```python
from build123d import *

# Parameters (mm, degrees)
SKETCH1_R                = 9.5
BOSS_EXTRUDE1_DEPTH      = 3
BOSS_EXTRUDE1_2_DEPTH    = 3
BOSS_EXTRUDE2_DEPTH      = 5
BOSS_EXTRUDE3_DEPTH      = 15.5
BOSS_EXTRUDE3_DEPTH_BACK = 1.5
BOSS_EXTRUDE4_DEPTH      = 8.5
BOSS_EXTRUDE4_DEPTH_BACK = 1.5
SKETCH1_5_R              = 10
SKETCH1_5_R_2            = 2.5
BOSS_EXTRUDE5_DEPTH      = 8.5
BOSS_EXTRUDE5_DEPTH_BACK = 1.5
SKETCH1_6_R              = 2.5
BOSS_EXTRUDE6_DEPTH      = 15.5
BOSS_EXTRUDE6_DEPTH_BACK = 1.5
SKETCH1_7_R              = 20
SKETCH1_7_R_2            = 15.5
CUT_EXTRUDE1_REACH       = 89.409
SKETCH8_W                = 16.25
SKETCH8_H                = 1.075
BOSS_EXTRUDE7_START      = 1.5
BOSS_EXTRUDE7_DEPTH      = 1.5


with BuildPart() as part:
    # Sketch1 → Boss-Extrude1 (new body)
    with BuildSketch(Plane(origin=(0, 0, 0), x_dir=(1, 0, 0), z_dir=(0, 1, 0))):
        with BuildLine():
            ThreePointArc((-30.156865167, -2.5), (-33.272749334, -10.963534337), (-39.790126097, -17.197629921))
            ThreePointArc((-39.790126097, -17.197629921), (-41.249487369, -19.543048034), (-40.173039204, -22.087056839))
            Line((-40.173039204, -22.087056839), (-14.241082593, -35.680284508))
            ThreePointArc((-14.241082593, -35.680284508), (-11.504148883, -36.255537388), (-9.482068, -34.323463137))
            ThreePointArc((-9.482068, -34.323463137), (-1.352594655, -27.591897876), (8.28370035, -31.898187034))
            ThreePointArc((8.28370035, -31.898187034), (10.418414325, -33.197109967), (12.796233312, -32.428877315))
            Line((12.796233312, -32.428877315), (28.974944097, -17.384928273))
            ThreePointArc((28.974944097, -17.384928273), (29.945946241, -15.076495792), (28.827477371, -12.835796554))
            ThreePointArc((28.827477371, -12.835796554), (27.255378579, -11.246023539), (26.082304527, -9.342665949))
            ThreePointArc((26.082304527, -9.342665949), (24.834057729, -6.000240645), (24.142507006, -2.5))
            Line((24.142507006, -2.5), (-30.156865167, -2.5))
        make_face()
        with Locations(Location((1, -14.5, 0), (0, 0, 270))):
            Circle(SKETCH1_R, mode=Mode.SUBTRACT)
    extrude(amount=BOSS_EXTRUDE1_DEPTH)



with BuildPart() as body_2:
    # Sketch1 → Boss-Extrude1 2 (new body)
    with BuildSketch(Plane(origin=(0, 0, 0), x_dir=(1, 0, 0), z_dir=(0, 1, 0))):
        with BuildLine():
            ThreePointArc((8.284210438, 31.898941402), (-1.363739049, 27.593425627), (-9.489477618, 34.345667337))
            ThreePointArc((-9.489477618, 34.345667337), (-11.573635866, 36.300800208), (-14.349825716, 35.623282637))
            Line((-14.349825716, 35.623282637), (-40.302516761, 22.019186222))
            ThreePointArc((-40.302516761, 22.019186222), (-41.273789994, 19.493443338), (-39.816532128, 17.213279237))
            ThreePointArc((-39.816532128, 17.213279237), (-33.281167386, 10.97636716), (-30.156865167, 2.5))
            Line((-30.156865167, 2.5), (24.142507006, 2.5))
            ThreePointArc((24.142507006, 2.5), (24.834057729, 6.000240645), (26.082304527, 9.342665949))
            ThreePointArc((26.082304527, 9.342665949), (27.255658523, 11.24637974), (28.828183508, 12.836364321))
            ThreePointArc((28.828183508, 12.836364321), (29.944640188, 15.02344116), (29.053717415, 17.311680053))
            Line((29.053717415, 17.311680053), (12.87474854, 32.355869082))
            ThreePointArc((12.87474854, 32.355869082), (10.472331387, 33.203871974), (8.284210438, 31.898941402))
        make_face()
        with Locations(Location((1, 14.5, 0), (0, 0, 270))):
            Circle(SKETCH1_R, mode=Mode.SUBTRACT)
    extrude(amount=BOSS_EXTRUDE1_2_DEPTH)


with BuildPart() as part_1:
    add(part.part)

    add(body_2.part)  # Boss-Extrude2 merges body 2
    # Sketch1_3 → Boss-Extrude2 (add)
    with BuildSketch(Plane(origin=(0, 0, 0), x_dir=(1, 0, 0), z_dir=(0, 1, 0))):
        with BuildLine():
            ThreePointArc((-39.790126097, -17.197629921), (-49.47057805, -19.992991582), (-59.285404172, -17.713872229))
            Line((-59.285404172, -17.713872229), (-4.642702086, -46.356936115))
            ThreePointArc((-4.642702086, -46.356936115), (-9.277844603, -41.231165974), (-9.482068, -34.323463137))
            ThreePointArc((-9.482068, -34.323463137), (-11.504148883, -36.255537388), (-14.241082593, -35.680284508))
            Line((-14.241082593, -35.680284508), (-40.173039204, -22.087056839))
            ThreePointArc((-40.173039204, -22.087056839), (-41.249487369, -19.543048034), (-39.790126097, -17.197629921))
        make_face()
        with BuildLine():
            ThreePointArc((10, -37.5), (9.167764123, -41.494008136), (6.809579802, -44.823224898))
            Line((6.809579802, -44.823224898), (41.707436105, -12.373076129))
            ThreePointArc((41.707436105, -12.373076129), (35.353639159, -15.0033493), (28.827477371, -12.835796554))
            ThreePointArc((28.827477371, -12.835796554), (29.945946241, -15.076495792), (28.974944097, -17.384928273))
            Line((28.974944097, -17.384928273), (12.796233312, -32.428877315))
            ThreePointArc((12.796233312, -32.428877315), (10.418414325, -33.197109967), (8.28370035, -31.898187034))
            ThreePointArc((8.28370035, -31.898187034), (9.561302304, -34.570580561), (10, -37.5))
        make_face()
        with BuildLine():
            Line((41.707436105, 12.373076129), (6.809579802, 44.823224898))
            ThreePointArc((6.809579802, 44.823224898), (9.167764123, 41.494008136), (10, 37.5))
            ThreePointArc((10, 37.5), (9.561435676, 34.571015908), (8.284210438, 31.898941402))
            ThreePointArc((8.284210438, 31.898941402), (10.472331387, 33.203871974), (12.87474854, 32.355869082))
            Line((12.87474854, 32.355869082), (29.053717415, 17.311680053))
            ThreePointArc((29.053717415, 17.311680053), (29.944640188, 15.02344116), (28.828183508, 12.836364321))
            ThreePointArc((28.828183508, 12.836364321), (35.354091909, 15.003333024), (41.707436105, 12.373076129))
        make_face()
        with BuildLine():
            ThreePointArc((-9.489477618, 34.345667337), (-9.273471314, 41.242022153), (-4.642702086, 46.356936115))
            Line((-4.642702086, 46.356936115), (-59.285404172, 17.713872229))
            ThreePointArc((-59.285404172, 17.713872229), (-49.4859203, 19.99339196), (-39.816532128, 17.213279237))
            ThreePointArc((-39.816532128, 17.213279237), (-41.273789994, 19.493443338), (-40.302516761, 22.019186222))
            Line((-40.302516761, 22.019186222), (-14.349825716, 35.623282637))
            ThreePointArc((-14.349825716, 35.623282637), (-11.573635866, 36.300800208), (-9.489477618, 34.345667337))
        make_face()
    extrude(amount=BOSS_EXTRUDE2_DEPTH)

    # Sketch1_4 → Boss-Extrude3 (add, two sides: drawn at the far end of the back side and taken through both)
    with BuildSketch(Plane(origin=(0, 0, 0), x_dir=(1, 0, 0), z_dir=(0, 1, 0)).offset(-BOSS_EXTRUDE3_DEPTH_BACK)):
        with BuildLine():
            Line((24.142507006, 2.5), (-30.156865167, 2.5))
            ThreePointArc((-30.156865167, 2.5), (-30.039254815, 1.252458251), (-30, 0))
            ThreePointArc((-30, 0), (-30.039254815, -1.252458251), (-30.156865167, -2.5))
            Line((-30.156865167, -2.5), (24.142507006, -2.5))
            ThreePointArc((24.142507006, -2.5), (24, 0), (24.142507006, 2.5))
        make_face()
    extrude(amount=BOSS_EXTRUDE3_DEPTH + BOSS_EXTRUDE3_DEPTH_BACK)

    # Sketch1_5 → Boss-Extrude4 (add, two sides: drawn at the far end of the back side and taken through both)
    # profile 1 of 2: a face of its own
    with BuildSketch(Plane(origin=(0, 0, 0), x_dir=(1, 0, 0), z_dir=(0, 1, 0)).offset(-BOSS_EXTRUDE4_DEPTH_BACK)):
        with Locations(Location((0, -37.5, 0), (0, 0, 270))):
            Circle(SKETCH1_5_R)
        with Locations(Location((0, -37.5, 0), (0, 0, 270))):
            Circle(SKETCH1_5_R_2, mode=Mode.SUBTRACT)
    # profile 2 of 2: a face of its own
    with BuildSketch(Plane(origin=(0, 0, 0), x_dir=(1, 0, 0), z_dir=(0, 1, 0)).offset(-BOSS_EXTRUDE4_DEPTH_BACK)):
        with Locations(Location((0, 37.5, 0), (0, 0, 270))):
            Circle(SKETCH1_5_R)
        with Locations(Location((0, 37.5, 0), (0, 0, 270))):
            Circle(SKETCH1_5_R_2, mode=Mode.SUBTRACT)
    extrude(amount=BOSS_EXTRUDE4_DEPTH + BOSS_EXTRUDE4_DEPTH_BACK)

    # Sketch1_6 → Boss-Extrude5 (add, two sides: drawn at the far end of the back side and taken through both)
    with BuildSketch(Plane(origin=(0, 0, 0), x_dir=(1, 0, 0), z_dir=(0, 1, 0)).offset(-BOSS_EXTRUDE5_DEPTH_BACK)):
        with BuildLine():
            ThreePointArc((26.082304527, -9.342665949), (35, -15.009699604), (43.917695473, -9.342665949))
            ThreePointArc((43.917695473, -9.342665949), (46, 0), (43.917695473, 9.342665949))
            ThreePointArc((43.917695473, 9.342665949), (35, 15.009699604), (26.082304527, 9.342665949))
            ThreePointArc((26.082304527, 9.342665949), (24, 0), (26.082304527, -9.342665949))
        make_face()
        with Locations(Location((35, 0, 0), (0, 0, 270))):
            Circle(SKETCH1_6_R, mode=Mode.SUBTRACT)
    extrude(amount=BOSS_EXTRUDE5_DEPTH + BOSS_EXTRUDE5_DEPTH_BACK)

    # Sketch1_7 → Boss-Extrude6 (add, two sides: drawn at the far end of the back side and taken through both)
    with BuildSketch(Plane(origin=(0, 0, 0), x_dir=(1, 0, 0), z_dir=(0, 1, 0)).offset(-BOSS_EXTRUDE6_DEPTH_BACK)):
        with Locations((-50, 0)):
            Circle(SKETCH1_7_R)
        with Locations(Location((-50, 0, 0), (0, 0, 270))):
            Circle(SKETCH1_7_R_2, mode=Mode.SUBTRACT)
    extrude(amount=BOSS_EXTRUDE6_DEPTH + BOSS_EXTRUDE6_DEPTH_BACK)

    # Sketch3 → Cut-Extrude1 (cut, up to next)
    with BuildSketch(Plane.XY.offset(2.5), mode=Mode.PRIVATE) as cut_extrude1_sk1:
        Polygon((-30.156865167, 15.5), (24.142507006, 8.5), (24.142507006, 15.5), align=None)
    cut_extrude1_tool1 = extrude(cut_extrude1_sk1.sketch, amount=-CUT_EXTRUDE1_REACH, mode=Mode.PRIVATE) & part_1.part
    add(cut_extrude1_tool1.solids().sort_by_distance((6.042716, 13.166667, 2.5))[0], mode=Mode.SUBTRACT)

    # Sketch8 → Cut-Revolve2 (revolve, cut)
    with BuildSketch(Plane.XY, mode=Mode.PRIVATE) as cut_revolve2_sk:
        with Locations((-41.953432584, 14.5375)):
            Rectangle(SKETCH8_W, SKETCH8_H)
        with Locations((-41.953432584, 2.9625)):
            Rectangle(SKETCH8_W, SKETCH8_H)
    revolve(cut_revolve2_sk.sketch.rotate(Axis((-50.078432584, 15.075, 0), (0, -1, 0)), 90), axis=Axis((-50.078432584, 15.075, 0), (0, -1, 0)), mode=Mode.SUBTRACT)

    # Sketch11 → Boss-Extrude7 (add)
    with BuildSketch(Plane.XZ.offset(BOSS_EXTRUDE7_START)):
        with BuildLine():
            Line((6.809579802, -44.823224898), (41.707436105, -12.373076129))
            ThreePointArc((41.707436105, -12.373076129), (33.124591223, -14.829515627), (26.082304527, -9.342665949))
            ThreePointArc((26.082304527, -9.342665949), (24.834057729, -6.000240645), (24.142507006, -2.5))
            Line((24.142507006, -2.5), (21.5, -2.5))
            Line((21.5, -2.5), (21.5, -11.421704032))
            ThreePointArc((21.5, -11.421704032), (21.250329237, -12.619906472), (20.542873941, -13.618671501))
            Line((20.542873941, -13.618671501), (7.921337912, -25.354943159))
            ThreePointArc((7.921337912, -25.354943159), (6.415668049, -26.109485774), (4.740696751, -25.933851362))
            ThreePointArc((4.740696751, -25.933851362), (-9.080647661, -28.909782421), (-11.285404172, -42.87490955))
            Line((-11.285404172, -42.87490955), (-4.642702086, -46.356936115))
            ThreePointArc((-4.642702086, -46.356936115), (-1.327368556, -27.58848686), (6.809579802, -44.823224898))
        make_face()
        with BuildLine():
            Line((41.707436105, 12.373076129), (6.809579802, 44.823224898))
            ThreePointArc((6.809579802, 44.823224898), (-1.327368556, 27.58848686), (-4.642702086, 46.356936115))
            Line((-4.642702086, 46.356936115), (-11.285404172, 42.87490955))
            ThreePointArc((-11.285404172, 42.87490955), (-9.080647661, 28.909782421), (4.740696751, 25.933851362))
            ThreePointArc((4.740696751, 25.933851362), (6.415668049, 26.109485774), (7.921337912, 25.354943159))
            Line((7.921337912, 25.354943159), (20.542873941, 13.618671501))
            ThreePointArc((20.542873941, 13.618671501), (21.250329237, 12.619906472), (21.5, 11.421704032))
            Line((21.5, 11.421704032), (21.5, 2.5))
            Line((21.5, 2.5), (24.142507006, 2.5))
            ThreePointArc((24.142507006, 2.5), (24.834057729, 6.000240645), (26.082304527, 9.342665949))
            ThreePointArc((26.082304527, 9.342665949), (33.124591223, 14.829515627), (41.707436105, 12.373076129))
        make_face()
    extrude(amount=-BOSS_EXTRUDE7_DEPTH)


solid = part_1.part
```
Check sheet for the modelled part. Datum: model origin and axes. Units: mm. A direction names the side the tool comes from. Round coordinates to 2 decimals unless told otherwise and drop trailing zeros. Loops run counter-clockwise (first coordinate to the right, second up) from the corner with the lowest first, then second, coordinate; pieces in that order, holes last. Notation, with made-up numbers: (61, 70) -> (73, 70) arc R19 ccw to (73, 94) -> close; hole circle Ø5 at (85, 23). An arc over 180 degrees is marked (long way). Write item = value, one per line. Start each with the question number.
1) Release check for a two-part mould opening along X. For faces 5 (the cylindrical face through (-8.274, 1.479, -16.559)), 6 (the flat face through (-37, 15.5, 9)) record: released by +X, released by -X, zero draft, split by the parting line, or undercut.
2) Thickness scan on probe 1 along Z at (x, y) = (-50, 6.25); probe 2 along Z at (x, y) = (14, 7.25); probe 3 along Y at (x, z) = (-27.5, -18.5). Record the ranges inside material, lowest first.
3) Sectioned sample at A-A, the plane z = 0. State how many separate pieces and enclosed holes the cut face has, plus the area to 3 significant figures.
4) Sectioned sample at B-B, the plane x = -62. Record the cut outline in (y, z) (3 decimals).
5) Sectioned sample at C-C, the plane x = -31.5. Record the cut outline in (y, z), plus the area to 3 significant figures.
6) Gauge pin test, flat ends, axial feed: pin 1 Ø4 at (y, z) = (7.5, -20) entering from +X; pin 2 Ø6 at (x, z) = (0, -37.5) entering from +Y; pin 3 Ø4 at (x, y) = (27.5, 11) entering from -Z; pin 4 Ø3 at (x, y) = (-18, 7) entering from -Z. Record the tip position at first contact, or that the pin passes through.
7) Set-up check for faces 1 (the flat face through (32, 8.5, 0)), 2 (the flat face through (-2, 8.5, -35)), 3 (the flat face through (14.32, -0.76, -19.405)), 4 (the flat face through (-56.2, 14, -14.4)): record each of +Z, -Z, +X, -X, +Y, -Y from which the full face is reachable in a straight line by a thin tool's end or side.
Results are:
q1.face_5 = undercut
q1.face_6 = zero draft
q2.probe_1 = -20 to -15.5, 15.5 to 20
q2.probe_2 = -2.5 to 2.5
q2.probe_3 = 0 to 3
q3.separate_pieces = 3
q3.enclosed_holes = 0
q3.area = 1,050 mm^2
q4.outline = (-1.5, -16) -> (15.5, -16) -> (15.5, -9.811) -> (15.075, -9.811) -> (15.075, -11.043) -> (14, -11.043) -> (14, -9.811) -> (3.5, -9.811) -> (3.5, -11.043) -> (2.425, -11.043) -> (2.425, -9.811) -> (-1.5, -9.811) -> close; (-1.5, 9.811) -> (2.425, 9.811) -> (2.425, 11.043) -> (3.5, 11.043) -> (3.5, 9.811) -> (14, 9.811) -> (14, 11.043) -> (15.075, 11.043) -> (15.075, 9.811) -> (15.5, 9.811) -> (15.5, 16) -> (-1.5, 16) -> close
q5.outline = (-1.5, -7.6) -> (0, -7.6) -> (0, -32.28) -> (5, -32.28) -> (5, -26.63) -> (3, -26.63) -> (3, -7.6) -> (15.5, -7.6) -> (15.5, 7.6) -> (3, 7.6) -> (3, 26.63) -> (5, 26.63) -> (5, 32.28) -> (0, 32.28) -> (0, 7.6) -> (-1.5, 7.6) -> close
q5.area = 429 mm^2
q6.pin_1 = -41.28
q6.pin_2 = 8.5
q6.pin_3 = through
q6.pin_4 = -2.5
q7.face_1 = +Z, -Z, +X, +Y
q7.face_2 = -Z, +X, -X, +Y
q7.face_3 = -Y
q7.face_4 = none
